Check sheet for the modelled part. Datum: model origin and axes. Units: mm. A direction names the side the tool comes from. Give positions to 0.01 mm unless a question says otherwise; leave off trailing zeros. Order: outer loops, then holes, each group sorted by start corner. A loop starts at its lowest first (then second) coordinate and runs counter-clockwise, first axis right, second up.
```python
from build123d import *

# Parameters (mm, degrees)
CROQUIS1_W                  = 85
CROQUIS1_H                  = 70
SALIENTE_EXTRUIR1_DEPTH     = 15
CROQUIS3_R                  = 4.15
CORTAR_EXTRUIR1_DEPTH       = 10
CORTAR_EXTRUIR2_DEPTH       = 1
SALIENTE_EXTRUIR4_START     = 10
SALIENTE_EXTRUIR4_DEPTH     = 10
CROQUIS9_W                  = 5.85
CROQUIS9_H                  = 10
SALIENTE_EXTRUIR5_DEPTH     = 9
CROQUIS10_W                 = 20
CROQUIS10_H                 = 10
SALIENTE_EXTRUIR6_DEPTH     = 1
CORTAR_EXTRUIR4_REACH       = 84.335
CROQUIS8_R                  = 1.75
CROQUIS12_W                 = 5.85
CROQUIS12_H                 = 10
CROQUIS12_R                 = 1.75
SALIENTE_EXTRUIR7_DEPTH     = 9
CROQUIS13_W                 = 20
CROQUIS13_H                 = 10
SALIENTE_EXTRUIR8_DEPTH     = 1
CROQUIS14_R                 = 1.75
CORTAR_EXTRUIR5_DEPTH       = 11
SALIENTE_EXTRUIR10_DEPTH    = 70
CROQUIS23_R                 = 5
CORTAR_EXTRUIR9_DEPTH       = 5
CROQUIS22_R                 = 5
CORTAR_EXTRUIR10_DEPTH      = 5
CORTAR_EXTRUIR11_DEPTH      = 59.576872569
CORTAR_EXTRUIR11_DEPTH_BACK = 59.576872569
CROQUIS24_R                 = 2.25
CROQUIS25_W                 = 12
CROQUIS25_H                 = 6
SALIENTE_EXTRUIR11_DEPTH    = 28
REDONDEO1_R                 = 4


with BuildPart() as part:
    # Croquis1 → Saliente-Extruir1 (new body)
    with BuildSketch(Plane(origin=(0, 0, 0), x_dir=(1, 0, 0), z_dir=(0, 1, 0))):
        Rectangle(CROQUIS1_W, CROQUIS1_H)
    extrude(amount=SALIENTE_EXTRUIR1_DEPTH)

    # Croquis3 → Cortar-Extruir1 (cut)
    with BuildSketch(Plane.XZ):
        with Locations(Location((-30.5, 0, 0), (0, 0, 270))):
            Circle(CROQUIS3_R)
        with Locations(Location((30.5, 0, 0), (0, 0, 270))):
            Circle(CROQUIS3_R)
    extrude(amount=-CORTAR_EXTRUIR1_DEPTH, mode=Mode.SUBTRACT)

    # Croquis4 → Cortar-Extruir2 (cut)
    with BuildSketch(Plane(origin=(0, 0, 0), x_dir=(-1, 0, 0), z_dir=(0, -1, 0))):
        Polygon((-3.109375, 6), (-2, 6), (-2, 0), (-2.538461538, 0), (-2.538461538, 5.384615385), (-3.461538462, 5.384615385), align=None)
        Polygon((1.506009615, 6), (2.615384615, 6), (2.615384615, 0), (2.076923077, 0), (2.076923077, 5.384615385), (1.153846154, 5.384615385), align=None)
    extrude(amount=-CORTAR_EXTRUIR2_DEPTH, mode=Mode.SUBTRACT)

    # Croquis5 → Saliente-Extruir4 (add)
    with BuildSketch(Plane.XZ.offset(SALIENTE_EXTRUIR4_START)):
        with BuildLine():
            Line((30.5, -4.15), (30.5, -10))
            ThreePointArc((30.5, -10), (20.5, 0), (30.5, 10))
            Line((30.5, 10), (30.5, 4.15))
            ThreePointArc((30.5, 4.15), (26.35, 0), (30.5, -4.15))
        make_face()
        with BuildLine():
            Line((-30.5, -10), (-30.5, -4.15))
            ThreePointArc((-30.5, -4.15), (-26.35, 0), (-30.5, 4.15))
            Line((-30.5, 4.15), (-30.5, 10))
            ThreePointArc((-30.5, 10), (-20.5, 0), (-30.5, -10))
        make_face()
    extrude(amount=-SALIENTE_EXTRUIR4_DEPTH)

    # Croquis9 → Saliente-Extruir5 (add)
    with BuildSketch(Plane(origin=(30.5, 0, 0), x_dir=(0, 0, -1), z_dir=(1, 0, 0))):
        with Locations((7.075, -5)):
            Rectangle(CROQUIS9_W, CROQUIS9_H)
        with Locations((-7.075, -5)):
            Rectangle(CROQUIS9_W, CROQUIS9_H)
    extrude(amount=-SALIENTE_EXTRUIR5_DEPTH)

    # Croquis10 → Saliente-Extruir6 (add)
    with BuildSketch(Plane.ZY.offset(-21.5)):
        with Locations((0, -5)):
            Rectangle(CROQUIS10_W, CROQUIS10_H)
    extrude(amount=SALIENTE_EXTRUIR6_DEPTH)

    # Croquis8 → Cortar-Extruir4 (cut, up to next)
    with BuildSketch(Plane(origin=(30.5, 0, 0), x_dir=(0, 0, -1), z_dir=(1, 0, 0)), mode=Mode.PRIVATE) as cortar_extruir4_sk1:
        with Locations((7.075, -4.609756337)):
            Circle(CROQUIS8_R)
    cortar_extruir4_tool1 = extrude(cortar_extruir4_sk1.sketch, amount=-CORTAR_EXTRUIR4_REACH, mode=Mode.PRIVATE) & part.part
    # Croquis8 → Cortar-Extruir4 (cut, up to next)
    with BuildSketch(Plane(origin=(30.5, 0, 0), x_dir=(0, 0, -1), z_dir=(1, 0, 0)), mode=Mode.PRIVATE) as cortar_extruir4_sk2:
        with Locations((-7.07, -4.609756337)):
            Circle(CROQUIS8_R)
    cortar_extruir4_tool2 = extrude(cortar_extruir4_sk2.sketch, amount=-CORTAR_EXTRUIR4_REACH, mode=Mode.PRIVATE) & part.part
    add(cortar_extruir4_tool1.solids().sort_by_distance((30.5, -4.609756, -7.075))[0], mode=Mode.SUBTRACT)
    add(cortar_extruir4_tool2.solids().sort_by_distance((30.5, -4.609756, 7.07))[0], mode=Mode.SUBTRACT)

    # Croquis12 → Saliente-Extruir7 (add)
    # profile 1 of 2: a face of its own
    with BuildSketch(Plane.ZY.offset(30.5)):
        with Locations((7.075, -5)):
            Rectangle(CROQUIS12_W, CROQUIS12_H)
        with Locations((7.07, -5)):
            Circle(CROQUIS12_R, mode=Mode.SUBTRACT)
    # profile 2 of 2: a face of its own
    with BuildSketch(Plane.ZY.offset(30.5)):
        with Locations((-7.075, -5)):
            Rectangle(CROQUIS12_W, CROQUIS12_H)
        with Locations((-7.07, -5)):
            Circle(CROQUIS12_R, mode=Mode.SUBTRACT)
    extrude(amount=-SALIENTE_EXTRUIR7_DEPTH)

    # Croquis13 → Saliente-Extruir8 (add)
    with BuildSketch(Plane(origin=(-21.5, 0, 0), x_dir=(0, 0, -1), z_dir=(1, 0, 0))):
        with Locations((0, -5)):
            Rectangle(CROQUIS13_W, CROQUIS13_H)
    extrude(amount=SALIENTE_EXTRUIR8_DEPTH)

    # Croquis14 → Cortar-Extruir5 (cut)
    with BuildSketch(Plane.ZY.offset(30.5)):
        with Locations((7.07, -5)):
            Circle(CROQUIS14_R)
        with Locations((-7.07, -5)):
            Circle(CROQUIS14_R)
    extrude(amount=-CORTAR_EXTRUIR5_DEPTH, mode=Mode.SUBTRACT)

    # Croquis15 → Saliente-Extruir10 (add, through all)
    with BuildSketch(Plane(origin=(0, 0, -35), x_dir=(-1, 0, 0), z_dir=(0, 0, -1))):
        Polygon((-26.5, 15), (-29.386751346, 20), (-8.386751346, 20), (-11.273502692, 15), align=None)
        Polygon((8.386751346, 20), (11.273502692, 15), (26.5, 15), (29.386751346, 20), align=None)
    extrude(amount=-SALIENTE_EXTRUIR10_DEPTH)

    # Croquis23 → Cortar-Extruir9 (cut)
    with BuildSketch(Plane(origin=(0, 15, 0), x_dir=(1, 0, 0), z_dir=(0, 1, 0))):
        with Locations(Location((-35.5, -25, 0), (0, 0, 270))):
            Circle(CROQUIS23_R)
    extrude(amount=-CORTAR_EXTRUIR9_DEPTH, mode=Mode.SUBTRACT)

    # Croquis22 → Cortar-Extruir10 (cut)
    with BuildSketch(Plane(origin=(0, 15, 0), x_dir=(1, 0, 0), z_dir=(0, 1, 0))):
        with Locations(Location((35.5, -25, 0), (0, 0, 270))):
            Circle(CROQUIS22_R)
    extrude(amount=-CORTAR_EXTRUIR10_DEPTH, mode=Mode.SUBTRACT)

    # Croquis24 → Cortar-Extruir11 (cut, two sides: drawn at the far end of the back side and taken through both)
    with BuildSketch(Plane(origin=(0, 10, 0), x_dir=(1, 0, 0), z_dir=(0, 1, 0)).offset(-CORTAR_EXTRUIR11_DEPTH_BACK)):
        with Locations(Location((-35.5, -25, 0), (0, 0, 270))):
            Circle(CROQUIS24_R)
        with Locations(Location((35.5, -25, 0), (0, 0, 270))):
            Circle(CROQUIS24_R)
    extrude(amount=CORTAR_EXTRUIR11_DEPTH + CORTAR_EXTRUIR11_DEPTH_BACK, mode=Mode.SUBTRACT)

    # Croquis25 → Saliente-Extruir11 (add)
    with BuildSketch(Plane.XZ):
        with Locations((-0.1, -23)):
            Rectangle(CROQUIS25_W, CROQUIS25_H)
    extrude(amount=SALIENTE_EXTRUIR11_DEPTH)

    # Redondeo1
    redondeo1_edges = [part.edges().sort_by_distance(p)[0] for p in [
        (5.9, 0, -23),
        (-0.1, 0, -20),
        (-6.1, 0, -23),
        (-0.1, 0, -26),
    ]]
    fillet(redondeo1_edges, radius=REDONDEO1_R)


solid = part.part
```
Q1. Draft check along X on faces 1 (the cylindrical face through (-33.603, 4.93, 26.21)), 2 (the flat face through (-30.5, -5, -9)), 3 (the flat face through (-26, -5, 10)). Enter one of: pulls with the +X half, pulls with the -X half, needs draft (parallel to the pull), parting line crosses it, or undercut.
Q2. Sectioned sample at A-A, the plane y = -9. Record the cut outline in (x, z).
Q3. Go/stop test with flat-tipped pins: P1, Ø4, axis at y = -22, z = -25, coming from the +X side; P2, Ø11, axis at x = -33, z = 23.5, coming from the +Y side; P3, Ø4, axis at y = -4.61, z = 7.07, coming from the +X side; P4, Ø6.5, axis at y = -6.5, z = -7.5, coming from the -X side. Record where each tip stops, or that it passes through.
Q4. Tool access check on faces 4 (the flat face through (-27.92, 17.46, -0.49)), 5 (the flat face through (0, 15, 0)), 6 (the cylindrical face through (25.57, -4.53, 8.82)), 7 (the flat face through (-30.5, -5, 5)). Record the directions out of +Z, -Z, +X, -X, +Y, -Y that give a thin tool (end or side, any length) a straight path to the whole face; none if there is none.
Q5. Sectioned sample at C-C, the plane y = 17. Record the cut outline in (x, z).
Q6. Material ranges on line 1 (X direction, y = 2, z = 25); line 2 (X direction, y = 11, z = 25); line 3 (X direction, y = -1.75, z = 0), recorded low to high.
Q7. Sectioned sample at D-D, the plane x = 7. Record the cut outline in (y, z) (3 decimals).
Q8. Sectioned sample at B-B, the plane z = 25. Record the cut outline in (x, y), plus the area to 3 significant figures.
Filled in:
1. face 1: undercut
1. face 2: pulls with the -X half
1. face 3: needs draft
2. outline: (-30.5, -10) - (-20.5, -10) - (-20.5, 10) - (-30.5, 10) - (-30.5, 4.15) arc R4.15 cw to (-30.5, -4.15) - close; (-6.1, -26) - (5.9, -26) - (5.9, -20) - (-6.1, -20) - close; (20.5, -10) - (30.5, -10) - (30.5, -4.15) arc R4.15 cw to (30.5, 4.15) - (30.5, 10) - (20.5, 10) - close
3. P1: stops at x = 5.9
3. P2: stops at y = 20
3. P3: stops at x = 30.5
3. P4: stops at x = -30.5
4. face 4: +Z, -Z, -X
4. face 5: +Z, -Z
4. face 6: +X
4. face 7: +Z, -Z, -X, -Y
5. outline: (-27.65, -35) - (-10.12, -35) - (-10.12, 35) - (-27.65, 35) - close; (10.12, -35) - (27.65, -35) - (27.65, 35) - (10.12, 35) - close
6. line 1: x = -42.5 to -37.75, -33.25 to 33.25, 37.75 to 42.5
6. line 2: x = -42.5 to -40.5, -30.5 to 30.5, 40.5 to 42.5
6. line 3: x = -26.35 to -20.5, 20.5 to 26.35
7. outline: (-1.245, -27.1) arc R4 cw to (0, -30) - (0, -35) - (15, -35) - (15, 35) - (0, 35) - (0, -16) arc R4 cw to (-1.245, -18.9) - close
8. outline: (-42.5, 0) - (-37.75, 0) - (-37.75, 10) - (-40.5, 10) - (-40.5, 15) - (-42.5, 15) - close; (-33.25, 0) - (33.25, 0) - (33.25, 10) - (30.5, 10) - (30.5, 15) - (26.5, 15) - (29.39, 20) - (8.39, 20) - (11.27, 15) - (-11.27, 15) - (-8.39, 20) - (-29.39, 20) - (-26.5, 15) - (-30.5, 15) - (-30.5, 10) - (-33.25, 10) - close; (37.75, 0) - (42.5, 0) - (42.5, 15) - (40.5, 15) - (40.5, 10) - (37.75, 10) - close
8. area: 1,270 mm2
